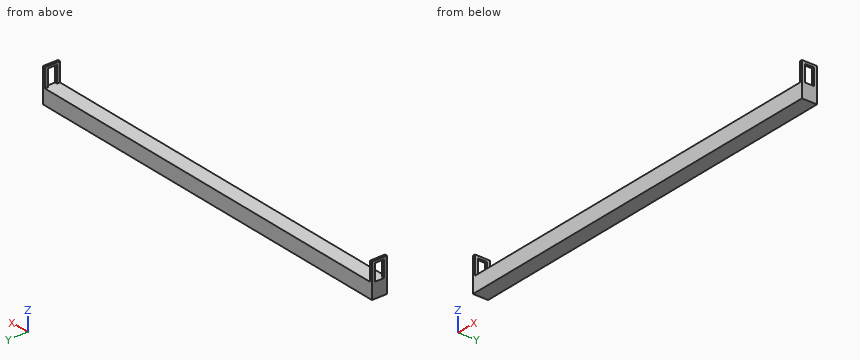
from build123d import *

# Parameters (mm, degrees)
SKETCH_W     = 53
SKETCH_H     = 2
PAD_DEPTH    = 2
SKETCH001_W  = 0.3
SKETCH001_H  = 2
PAD001_DEPTH = 2.5
SKETCH002_W  = 1.2
SKETCH002_H  = 2.2
POCKET_DEPTH = 0.3


with BuildPart() as part:
    # Sketch → Pad (new body)
    with BuildSketch(Plane.XY):
        Rectangle(SKETCH_W, SKETCH_H)
    extrude(amount=PAD_DEPTH)

    # Sketch001 (on Face6 of Pad) → Pad001 (join)
    with BuildSketch(Plane.XY.offset(2)):
        with Locations((-26.35, 0)):
            Rectangle(SKETCH001_W, SKETCH001_H)
    pad001 = extrude(amount=PAD001_DEPTH)

    # Sketch002 (on Face8 of Pad001) → Pocket (cut)
    with BuildSketch(Plane(origin=(-26.5, 0, 0), x_dir=(0, -1, 0), z_dir=(-1, 0, 0))):
        with Locations((0, 3.1)):
            Rectangle(SKETCH002_W, SKETCH002_H)
    pocket = extrude(amount=-POCKET_DEPTH, mode=Mode.SUBTRACT)

    # Mirrored: Pad001 across Sketch001 V_Axis
    add(pad001.mirror(Plane(origin=(0, 0, 2), x_dir=(0, 0, 1), z_dir=(1, 0, 0))))

    # Mirrored001: Pocket across YZ
    add(pocket.mirror(Plane.YZ), mode=Mode.SUBTRACT)


solid = part.part
Input: part model. Units: mm. Frame: model coordinates. Coordinates: 2 decimals unless noted, no trailing zeros. Loops run counter-clockwise (first coordinate to the right, second up) from the corner with the lowest first, then second, coordinate; pieces in that order, holes last.
Q1. Contact query for flat-ended pins moving along their axis: pin 1 (0.6 mm diameter, centred on x = -11, y = -0.5, fed in from +Z); pin 2 (0.6 mm diameter, centred on y = 0, z = 2.5, fed in from +X). Output: stop coordinate, or through.
Q2. Cut plane A-A (y = 0.15). Output: boundary loops of the cut face in (x, z), then the cut area to 3 significant figures.
Q3. Cut plane C-C (x = -6). Output: boundary loops of the cut face in (y, z).
Q4. Cut plane B-B (z = 2.65). Output: boundary loops of the cut face in (x, y).
Q5. Material intervals for line 1 (Z direction, x = 6, y = -0.05); line 2 (X direction, y = -0.7, z = 3.9), sorted ascending.
Working result:
1. pin 1: stops at z = 2
1. pin 2: passes through
2. outline: (-26.5, 0) - (26.5, 0) - (26.5, 2) - (-26.5, 2) - close; (-26.5, 4.2) - (-26.2, 4.2) - (-26.2, 4.5) - (-26.5, 4.5) - close; (26.2, 4.2) - (26.5, 4.2) - (26.5, 4.5) - (26.2, 4.5) - close
2. area: 106 mm2
3. outline: (-1, 0) - (1, 0) - (1, 2) - (-1, 2) - close
4. outline: (-26.5, -1) - (-26.2, -1) - (-26.2, -0.6) - (-26.5, -0.6) - close; (-26.5, 0.6) - (-26.2, 0.6) - (-26.2, 1) - (-26.5, 1) - close; (26.2, -1) - (26.5, -1) - (26.5, -0.6) - (26.2, -0.6) - close; (26.2, 0.6) - (26.5, 0.6) - (26.5, 1) - (26.2, 1) - close
5. line 1: z = 0 to 2
5. line 2: x = -26.5 to -26.2, 26.2 to 26.5
